Geometry: final body of the model. Coordinates: model frame, mm. Face numbers are marked on the shaded views. A direction names the side the tool comes from. Coordinates: 2 decimals unless noted, no trailing zeros. Loops run counter-clockwise (first coordinate to the right, second up) from the corner with the lowest first, then second, coordinate; pieces in that order, holes last. Notation, with made-up numbers: (85, 63.25) - (96, 63.25) arc R28 ccw to (96, 92.25) - close; hole circle Ø10 at (31.25, 49.25). An arc over 180 degrees is marked (long way). Return JSON: item names as keys, results as strings.
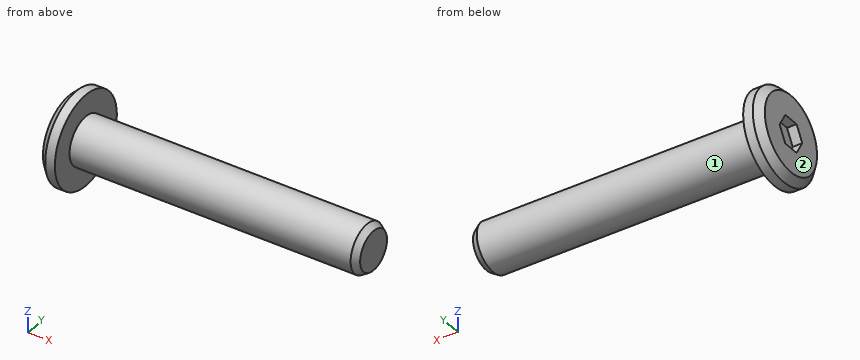
from build123d import *

# Parameters (mm, degrees)
CUT_EXTRUDE1_DEPTH = 1
CHAMFER1_SIZE      = 0.75


with BuildPart() as part:
    # Sketch1 → Revolve1 (revolve)
    with BuildSketch(Plane.XY):
        Polygon((31.75, 0), (31.75, 2.057236169), (31.055, 2.5), (1.75, 2.5), (1.75, 4.75), (0, 4.75), (0, 0), align=None)
    revolve(axis=Axis((0, 0, 0), (1, 0, 0)))

    # Sketch5 → Cut-Extrude1 (cut)
    with BuildSketch(Plane.ZY):
        Polygon((1.5, -0.866025404), (1.5, 0.866025404), (0, 1.732050808), (-1.5, 0.866025404), (-1.5, -0.866025404), (0, -1.732050808), align=None)
    extrude(amount=-CUT_EXTRUDE1_DEPTH, mode=Mode.SUBTRACT)

    # Chamfer1
    chamfer1_edges = [part.edges().sort_by_distance(p)[0] for p in [
        (0, -4.75, 0),
    ]]
    chamfer(chamfer1_edges, length=CHAMFER1_SIZE)


solid = part.part
Item 1: First-contact query: pin 1 Ø4 at (x, z) = (18.5, 1) entering from -Y; pin 2 Ø1.5 at (x, y) = (28.5, 3) entering from -Z; pin 3 Ø1.5 at (x, y) = (7.5, 3) entering from +Z. Flat tips, straight axial feed; report the tip coordinate or a pass-through.
Worked out:
{"pin 1": "y = -2.5", "pin 2": "z = -1.09", "pin 3": "z = 1.09"}
Item 2: Section query B-B, the plane x = 10. Return loops of the section in (y, z), and give its area (3 significant figures).
Worked out:
{"outline": "circle Ø5 at (0, 0)", "area": "19.6 mm^2"}
Item 3: Reachability of the marked faces 1 and 2 from +Z, -Z, +X, -X, +Y, -Y: full face, straight path, thin tool, end or side. Return the list, or none.
Worked out:
{"face 1": "+X", "face 2": "+Z, -Z, -X, +Y, -Y"}
Item 4: Section query A-A, the plane y = 0. Return loops of the section in (x, z) (3 decimals), and give its area (3 significant figures).
Worked out:
{"outline": "(0, -4) - (0.75, -4.75) - (1.75, -4.75) - (1.75, -2.5) - (31.055, -2.5) - (31.75, -2.057) - (31.75, 2.057) - (31.055, 2.5) - (1.75, 2.5) - (1.75, 4.75) - (0.75, 4.75) - (0, 4) - (0, 1.5) - (1, 1.5) - (1, -1.5) - (0, -1.5) - close", "area": "163 mm^2"}
Item 5: Ray query, probe 1 along X at (y, z) = (1.5, -2.25); probe 2 along Y at (x, z) = (20.5, -2); probe 3 along X at (y, z) = (0.5, 0). Return the intervals inside material, ascending. Write a range as from..to.
Worked out:
{"probe 1": "0..1.75", "probe 2": "-1.5..1.5", "probe 3": "1..31.75"}
